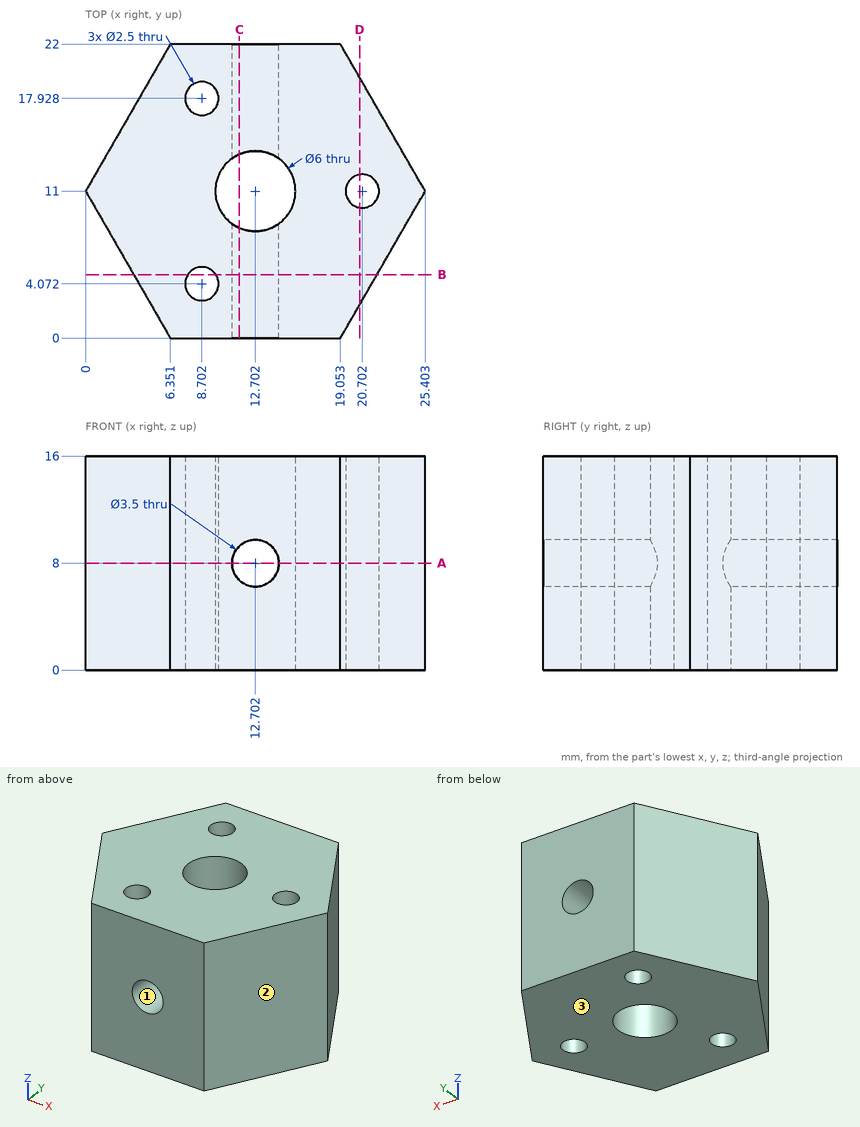
Answer from the drawing. Dimensions are ordinates in mm from the lowest x, y and z of the part. Round coordinates to 2 decimals unless told otherwise and drop trailing zeros. Loops run counter-clockwise (first coordinate to the right, second up) from the corner with the lowest first, then second, coordinate; pieces in that order, holes last.
Q1. Section A-A on z = 8 is taken. Write down the section's boundary in (x, y).
Q2. Each of these flat-tipped pins is pushed along its axis until it touches: pin 1 (3 mm diameter, centred on x = 2.5, z = 11, fed in from -Y); pin 2 (4 mm diameter, centred on x = 3, z = 3.5, fed in from +Y); pin 3 (5 mm diameter, centred on x = 12, y = 13, fed in from +Z). Where does it stop, or does it pass through?
Q3. Section B-B on y = 4.75 is taken. Give the number of separate pieces and of enclosed holes in the cut face, and give its area (3 significant figures).
Q4. Section D-D on x = 20.5 is taken. Write down the section's boundary in (y, z), and give its area (3 significant figures).
Q5. Section C-C on x = 11.5 is taken. Write down the section's boundary in (y, z).
Q6. Consider probe 1 along Y at (x, z) = (7.75, 1) (1 decimal); probe 2 along X at (y, z) = (18.5, 1) (1 decimal); probe 3 along Y at (x, z) = (14.5, 8.5). Determine where each line is inside the solid, lowest interval first.
Q7. Determine the mould class of the marked faces 1, 2 and 3 for opening direction Z: released by +Z, released by -Z, zero draft, split by the parting line, or undercut.
Output:
1. outline: (0, 11) - (6.35, 0) - (10.95, 0) - (10.95, 8.56) arc R3 cw to (10.95, 13.44) - (10.95, 22) - (6.35, 22) - close; (14.45, 0) - (19.05, 0) - (25.4, 11) - (19.05, 22) - (14.45, 22) - (14.45, 13.44) arc R3 cw to (14.45, 8.56) - close; hole circle Ø2.5 at (8.7, 4.07); hole circle Ø2.5 at (8.7, 17.93); hole circle Ø2.5 at (20.7, 11)
2. pin 1: stops at y = 4.07
2. pin 2: stops at y = 19.66
2. pin 3: stops at z = 16
3. separate pieces: 2
3. enclosed holes: 1
3. area: 248 mm2
4. outline: (2.51, 0) - (9.77, 0) - (9.77, 16) - (2.51, 16) - close; (12.23, 0) - (19.49, 0) - (19.49, 16) - (12.23, 16) - close
4. area: 232 mm2
5. outline: (0, 0) - (8.25, 0) - (8.25, 6.73) - (0, 6.73) - close; (0, 9.27) - (8.25, 9.27) - (8.25, 16) - (0, 16) - close; (13.75, 0) - (22, 0) - (22, 6.73) - (13.75, 6.73) - close; (13.75, 9.27) - (22, 9.27) - (22, 16) - (13.75, 16) - close
6. probe 1: y = 0 to 3.3, 4.9 to 17.1, 18.7 to 22
6. probe 2: x = 4.3 to 7.6, 9.8 to 21.1
6. probe 3: y = 0 to 8.6, 13.4 to 22
7. face 1: undercut
7. face 2: zero draft
7. face 3: released by -Z
